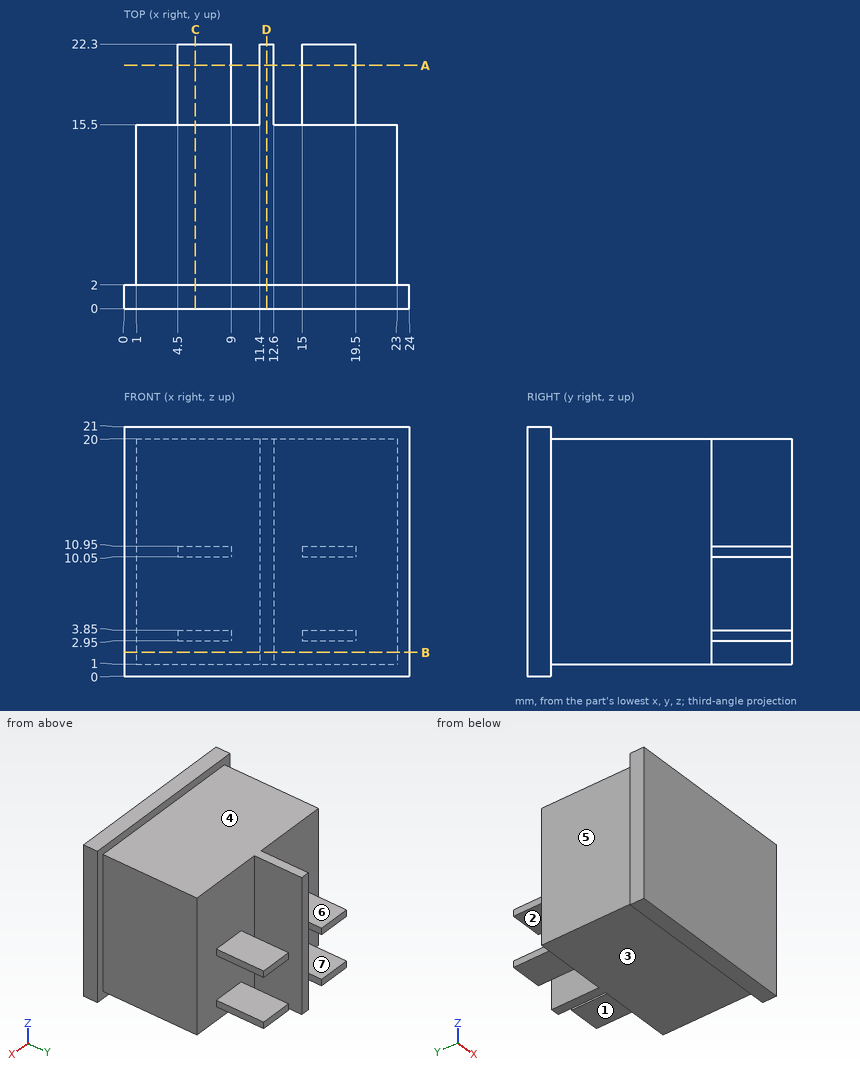
Here's the drawing with two shaded views (mm, measured from the low corner). I have some questions. A direction names the side the tool comes from. Give positions to 0.01 mm unless a question says otherwise; leave off trailing zeros. Loops run counter-clockwise (first coordinate to the right, second up) from the corner with the lowest first, then second, coordinate; pieces in that order, holes last. Notation, with made-up numbers: (1.25, 15.25) -> (14.25, 15.25) arc R16 cw to (14.25, 36.25) -> close; hole circle Ø4 at (32, 38). An arc over 180 degrees is marked (long way). Use one line per item in the form item = value.
1) If we section it at D-D (x = 12): Please give me the cut outline in (y, z), plus the area to 3 significant figures.
Answers:
outline = (0, 0) -> (2, 0) -> (2, 1) -> (22.3, 1) -> (22.3, 20) -> (2, 20) -> (2, 21) -> (0, 21) -> close
area = 428 mm²
2) For the marked faces 1, 2, 3 and 4, which set-ups out of +Z, -Z, +X, -X, +Y, -Y let a thin tool reach every point of the face, with its end or its side?
Answers:
face_1 = -Z, +X, +Y
face_2 = -X, +Y
face_3 = -Z, +X, -X, +Y
face_4 = +Z, +X, -X, +Y
3) I need wall thicknesses on line 1 along Z through (x, y) = (15.25, 21.25); line 2 along Y through (x, z) = (7.5, 1.25); line 3 along Z through (x, y) = (14, 4.5). Which ranges of each line are inside material? Lowest first, please.
Answers:
line_1 = 2.95 to 3.85, 10.05 to 10.95
line_2 = 0 to 15.5
line_3 = 1 to 20
4) If we section it at A-A (y = 20.5): Please give me the cut outline in (x, z), plus the area to 3 significant figures.
Answers:
outline = (4.5, 2.95) -> (9, 2.95) -> (9, 3.85) -> (4.5, 3.85) -> close; (4.5, 10.05) -> (9, 10.05) -> (9, 10.95) -> (4.5, 10.95) -> close; (11.4, 1) -> (12.6, 1) -> (12.6, 20) -> (11.4, 20) -> close; (15, 2.95) -> (19.5, 2.95) -> (19.5, 3.85) -> (15, 3.85) -> close; (15, 10.05) -> (19.5, 10.05) -> (19.5, 10.95) -> (15, 10.95) -> close
area = 39.0 mm²
5) If we section it at B-B (z = 2): Please give me the cut outline in (x, y).
Answers:
outline = (0, 0) -> (24, 0) -> (24, 2) -> (23, 2) -> (23, 15.5) -> (12.6, 15.5) -> (12.6, 22.3) -> (11.4, 22.3) -> (11.4, 15.5) -> (1, 15.5) -> (1, 2) -> (0, 2) -> close
6) We'd pull the mould along Z, two halves only. Please class the marked faces 5, 6 and 7: released by +Z, released by -Z, zero draft, split by the parting line, or undercut.
Answers:
face_5 = zero draft
face_6 = released by +Z
face_7 = undercut
7) Will these pins go through, and if not, where does the flat tip stop? pin 1 (1.3 mm diameter, centred on x = 18, y = 18.5, fed in from -Z); pin 2 (12 mm diameter, centred on x = 14, z = 11.5, fed in from +Y); pin 3 (0.7 mm diameter, centred on y = 19, z = 10.5, fed in from -X); pin 4 (1.3 mm diameter, centred on x = 6, y = 19, fed in from +Z).
Answers:
pin_1 = 2.95
pin_2 = 22.3
pin_3 = 4.5
pin_4 = 10.95
8) If we section it at C-C (x = 6): Please give me the cut outline in (y, z), plus the area to 3 significant figures.
Answers:
outline = (0, 0) -> (2, 0) -> (2, 1) -> (15.5, 1) -> (15.5, 2.95) -> (22.3, 2.95) -> (22.3, 3.85) -> (15.5, 3.85) -> (15.5, 10.05) -> (22.3, 10.05) -> (22.3, 10.95) -> (15.5, 10.95) -> (15.5, 20) -> (2, 20) -> (2, 21) -> (0, 21) -> close
area = 311 mm²
